Input: part model. Units: mm. Frame: model coordinates. Coordinates: 2 decimals unless noted, no trailing zeros. Order: outer loops, then holes, each group sorted by start corner. A loop starts at its lowest first (then second) coordinate and runs counter-clockwise, first axis right, second up. Notation, with made-up numbers: (-32.5, 81.25) - (-12.5, 81.25) arc R18 ccw to (-12.5, 88.25) - close; hole circle Ø8 at (-31.75, 71.5). An arc over 180 degrees is marked (long way). Answer as CSV lines item,"result". Start each with the question number.
Item 1: Section D-D (z = 0.8). State how many separate pieces and enclosed holes the cut face has, and give its area (3 significant figures).
Item 2: Section A-A (x = -21). Output: boundary loops of the cut face in (y, z).
Item 3: First-contact query: pin 1 (1.5 mm diameter, centred on y = 58, z = 1, fed in from -X); pin 2 (1 mm diameter, centred on y = 31, z = 2.5, fed in from -X); pin 3 (1.5 mm diameter, centred on x = -28.5, z = 1.5, fed in from -Y); pin 4 (1.5 mm diameter, centred on x = 15, z = 2, fed in from -Y). Flat tips, straight axial feed; report the tip coordinate or a pass-through.
Item 4: Section B-B (y = 33.5). Output: boundary loops of the cut face in (x, z).
Item 5: Section C-C (y = 48.5). Output: boundary loops of the cut face in (x, z).
Item 6: Material intervals for line 1 along Y through (x, z) = (13, 2.45); line 2 along X through (y, z) = (44.5, 1.65); line 3 along X through (y, z) = (45, 0.25), sorted ascending.
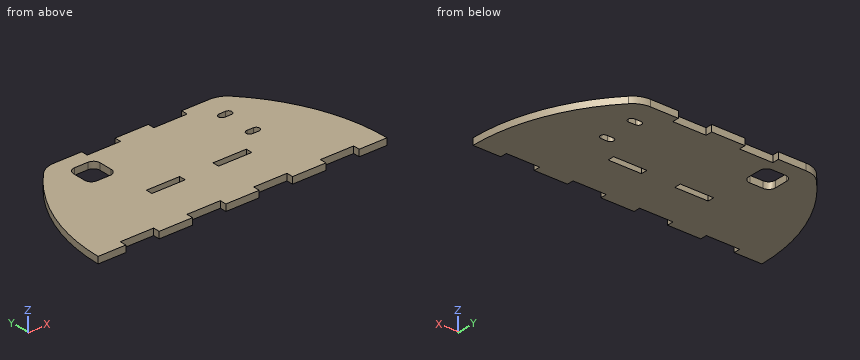
from build123d import *

# Parameters (mm, degrees)
BOSS_EXTRUDE1_DEPTH = 3
SKETCH2_W           = 15
SKETCH2_H           = 3
CUT_EXTRUDE1_DEPTH  = 89.509886453
CUT_EXTRUDE2_DEPTH  = 89.509886453
CUT_EXTRUDE3_DEPTH  = 89.509886453


with BuildPart() as part:
    # Sketch1 → Boss-Extrude1 (new body)
    with BuildSketch(Plane.XY):
        with BuildLine():
            Line((35, 60), (-35, 60))
            ThreePointArc((-35, 60), (-38.939192986, 59.1914503), (-42.24137931, 56.896551724))
            ThreePointArc((-42.24137931, 56.896551724), (-59.099326998, 30.639730799), (-65, 0))
            Line((-65, 0), (65, 0))
            ThreePointArc((65, 0), (59.099326998, 30.639730799), (42.24137931, 56.896551724))
            ThreePointArc((42.24137931, 56.896551724), (38.939192986, 59.1914503), (35, 60))
        make_face()
    extrude(amount=BOSS_EXTRUDE1_DEPTH)

    # Sketch2 → Cut-Extrude1 (cut, through all)
    with BuildSketch(Plane.XY.offset(3)):
        with Locations((-15, 58.5)):
            Rectangle(SKETCH2_W, SKETCH2_H)
        with Locations((-45, 1.5)):
            Rectangle(SKETCH2_W, SKETCH2_H)
        with Locations((-15, 1.5)):
            Rectangle(SKETCH2_W, SKETCH2_H)
        with Locations((-15, 23.5)):
            Rectangle(SKETCH2_W, SKETCH2_H)
    cut_extrude1 = extrude(amount=-CUT_EXTRUDE1_DEPTH, mode=Mode.SUBTRACT)

    # Mirror1: Cut-Extrude1 across plane
    add(cut_extrude1.mirror(Plane(origin=(0, 0, 0), x_dir=(0, 0, 1), z_dir=(1, 0, 0))), mode=Mode.SUBTRACT)

    # Sketch3 → Cut-Extrude2 (cut, through all)
    with BuildSketch(Plane.XY.offset(3)):
        with BuildLine():
            Line((-31.5, 53), (-25.5, 53))
            ThreePointArc((-25.5, 53), (-23.378679656, 52.121320344), (-22.5, 50))
            Line((-22.5, 50), (-22.5, 44))
            ThreePointArc((-22.5, 44), (-23.378679656, 41.878679656), (-25.5, 41))
            Line((-25.5, 41), (-31.5, 41))
            ThreePointArc((-31.5, 41), (-33.621320344, 41.878679656), (-34.5, 44))
            Line((-34.5, 44), (-34.5, 50))
            ThreePointArc((-34.5, 50), (-33.621320344, 52.121320344), (-31.5, 53))
        make_face()
    extrude(amount=-CUT_EXTRUDE2_DEPTH, mode=Mode.SUBTRACT)

    # Sketch4 → Cut-Extrude3 (cut, through all)
    with BuildSketch(Plane.XY.offset(3)):
        with BuildLine():
            Line((31, 50), (34, 50))
            ThreePointArc((34, 50), (35.5, 48.5), (34, 47))
            Line((34, 47), (31, 47))
            ThreePointArc((31, 47), (29.5, 48.5), (31, 50))
        make_face()
        with BuildLine():
            Line((31, 35), (34, 35))
            ThreePointArc((34, 35), (35.5, 33.5), (34, 32))
            Line((34, 32), (31, 32))
            ThreePointArc((31, 32), (29.5, 33.5), (31, 35))
        make_face()
    extrude(amount=-CUT_EXTRUDE3_DEPTH, mode=Mode.SUBTRACT)


solid = part.part
Determined:
1,separate pieces,"1"
1,enclosed holes,"5"
1,area,"6,310 mm^2"
2,outline,"(3, 0) - (22, 0) - (22, 3) - (3, 3) - close; (25, 0) - (57, 0) - (57, 3) - (25, 3) - close"
3,pin 1,"stops at x = -41.89"
3,pin 2,"stops at x = -59.16"
3,pin 3,"stops at y = 0"
3,pin 4,"stops at y = 3"
4,outline,"(-57.89, 0) - (29.5, 0) - (29.5, 3) - (-57.89, 3) - close; (35.5, 0) - (57.89, 0) - (57.89, 3) - (35.5, 3) - close"
5,outline,"(-49.24, 0) - (-34.5, 0) - (-34.5, 3) - (-49.24, 3) - close; (-22.5, 0) - (29.5, 0) - (29.5, 3) - (-22.5, 3) - close; (35.5, 0) - (49.24, 0) - (49.24, 3) - (35.5, 3) - close"
6,line 1,"y = 3 to 22, 25 to 57"
6,line 2,"x = -51.97 to -34.5, -22.5 to 51.97"
6,line 3,"x = -51.65 to -34.5, -22.5 to 51.65"
